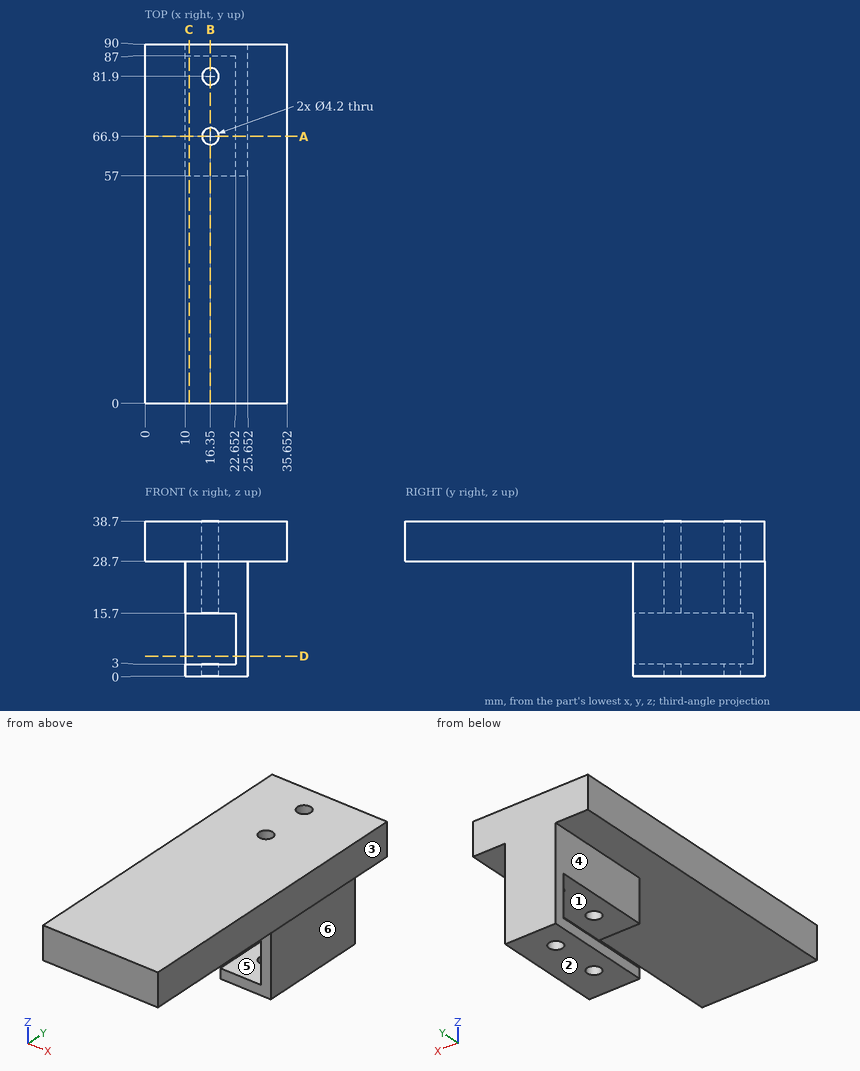
Here's the drawing with two shaded views (mm, measured from the low corner). I have some questions. A direction names the side the tool comes from. Give positions to 0.01 mm unless a question says otherwise; leave off trailing zeros. Write each loop counter-clockwise with the first axis right and the second up, starting at its lowest first coordinate (ties: lowest second). Pieces come first, ordered by that corner, then holes. Notation, with made-up numbers: (-7, -39.75) -> (46, -39.75) arc R12 ccw to (46, -16.75) -> close; hole circle Ø2 at (18, -22.5). An arc over 180 degrees is marked (long way). Answer as a JSON object with one key per item and string values. Group by question number.
Item 1: Suppose I cut it at D-D (z = 5). Please give me the cut outline in (x, y), plus the area to 3 significant figures.
Item 2: Suppose I cut it at A-A (y = 66.9). Please give me the cut outline in (x, z).
Item 3: For the marked faces 4, 5 and 6, which set-ups out of +Z, -Z, +X, -X, +Y, -Y let a thin tool reach every point of the face, with its end or its side?
Item 4: Suppose I cut it at B-B (x = 16.35). Please give me the cut outline in (y, z).
Item 5: Suppose I cut it at C-C (x = 11). Please give me the cut outline in (y, z).
Item 6: We'd pull the mould along Z, two halves only. Please class the marked faces 1, 2 and 3: +Z half, -Z half, draft (parallel to the pull), parting line (faces both ways), or undercut.
Item 7: Please list where these lines run through material, in increasing order: line 1 (Y direction, x = 16.5, z = 21) (1 decimal); line 2 (Y direction, x = 16.35, z = 29.25); line 3 (Z direction, x = 32, y = 60.5). Write a range as [from, to].
Item 8: I'm going to push flat-ended pins straight in: P1, Ø6.5, axis at x = 16.35, y = 66.9, coming from the +Z side; P2, Ø4, axis at x = 14.5, z = 12, coming from the -Y side; P3, Ø12, axis at x = 17, z = 4, coming from the -Y side; P4, Ø8.5, axis at y = 79.5, z = 15.5, coming from the +X side. Where does each tip first touch, or does it pass through?
Findings:
{
 "1": {"outline": "(10, 87) -> (22.65, 87) -> (22.65, 57) -> (25.65, 57) -> (25.65, 90) -> (10, 90) -> close", "area": "137 mm²"},
 "2": {"outline": "(0, 28.7) -> (10, 28.7) -> (10, 15.7) -> (14.25, 15.7) -> (14.25, 38.7) -> (0, 38.7) -> close; (10, 0) -> (14.25, 0) -> (14.25, 3) -> (10, 3) -> close; (18.45, 0) -> (25.65, 0) -> (25.65, 28.7) -> (35.65, 28.7) -> (35.65, 38.7) -> (18.45, 38.7) -> (18.45, 15.7) -> (22.65, 15.7) -> (22.65, 3) -> (18.45, 3) -> close"},
 "3": {"face 4": "-Z, -X, +Y, -Y", "face 5": "-X, -Y", "face 6": "-Z, +X, +Y, -Y"},
 "4": {"outline": "(0, 28.7) -> (57, 28.7) -> (57, 15.7) -> (64.8, 15.7) -> (64.8, 38.7) -> (0, 38.7) -> close; (57, 0) -> (64.8, 0) -> (64.8, 3) -> (57, 3) -> close; (69, 0) -> (79.8, 0) -> (79.8, 3) -> (69, 3) -> close; (69, 15.7) -> (79.8, 15.7) -> (79.8, 38.7) -> (69, 38.7) -> close; (84, 0) -> (90, 0) -> (90, 38.7) -> (84, 38.7) -> (84, 15.7) -> (87, 15.7) -> (87, 3) -> (84, 3) -> close"},
 "5": {"outline": "(0, 28.7) -> (57, 28.7) -> (57, 15.7) -> (87, 15.7) -> (87, 3) -> (57, 3) -> (57, 0) -> (90, 0) -> (90, 38.7) -> (0, 38.7) -> close"},
 "6": {"face 1": "undercut", "face 2": "-Z half", "face 3": "draft"},
 "7": {"line 1": "y = [57, 64.8], [69, 79.8], [84, 90]", "line 2": "y = [0, 64.8], [69, 79.8], [84, 90]", "line 3": "z = [28.7, 38.7]"},
 "8": {"P1": "stops at z = 38.7", "P2": "stops at y = 87", "P3": "stops at y = 57", "P4": "stops at x = 25.65"}
}
